from build123d import *

# Parameters (mm, degrees)
REVOLVE1_ANGLE     = 180
SKETCH3_R          = 1
CUT_EXTRUDE1_DEPTH = 2.5


with BuildPart() as part:
    # Sketch1 → Revolve1 (revolve)
    with BuildSketch(Plane(origin=(0, 0, 0), x_dir=(1, 0, 0), z_dir=(0, 1, 0))):
        with BuildLine():
            Line((0, 18.516950365), (120, 9.258475183))
            ThreePointArc((120, 9.258475183), (126.546730585, 6.546730585), (129.258475183, 0))
            Line((129.258475183, 0), (126, 0))
            ThreePointArc((126, 0), (124.242640687, 4.242640687), (120, 6))
            Line((120, 6), (0, 14))
            ThreePointArc((0, 14), (-9.899494937, 9.899494937), (-14, 0))
            Line((-14, 0), (-18.516950365, 0))
            ThreePointArc((-18.516950365, 0), (-13.09346117, 13.09346117), (0, 18.516950365))
        make_face()
    revolve(axis=Axis((-18.516950365, 0, 0), (1, 0, 0)), revolution_arc=REVOLVE1_ANGLE)

    # Sketch3 → Cut-Extrude1 (cut)
    with BuildSketch(Plane.XZ):
        with Locations(Location((-16, 0, 0), (0, 0, 270))):
            Circle(SKETCH3_R)
        with Locations(Location((0, 16, 0), (0, 0, 270))):
            Circle(SKETCH3_R)
        with Locations(Location((0, -16, 0), (0, 0, 270))):
            Circle(SKETCH3_R)
        with Locations(Location((127.5, 0, 0), (0, 0, 270))):
            Circle(SKETCH3_R)
    extrude(amount=-CUT_EXTRUDE1_DEPTH, mode=Mode.SUBTRACT)


solid = part.part
Can you work these out from the model? Positions are in its coordinate system, mm. A direction names the side the tool comes from. Give positions to 0.01 mm unless a question says otherwise; leave off trailing zeros. Loops run counter-clockwise (first coordinate to the right, second up) from the corner with the lowest first, then second, coordinate; pieces in that order, holes last. Notation, with made-up numbers: (16, -38.75) -> (50, -38.75) arc R24 ccw to (50, -20.75) -> close; hole circle Ø10 at (58.5, -22). An arc over 180 degrees is marked (long way). Return JSON: item names as keys, results as strings.
Q1. I want a section at B-B, the plane x = 15. List the corners of the cut face in (y, z) for me.
Checks:
{"outline": "(0, -17.36) arc R17.36 ccw to (0, 17.36) -> (0, 13) arc R13 cw to (0, -13) -> close"}
Q2. I want a section at A-A, the plane x = 87. List the corners of the cut face in (y, z) for me, then the cut area to 3 significant figures.
Checks:
{"outline": "(0, -11.8) arc R11.8 ccw to (0, 11.8) -> (0, 8.2) arc R8.2 cw to (0, -8.2) -> close", "area": "113 mm2"}
Q3. For pin 1 Ø1 at (x, y) = (80.5, 5) entering from +Z; pin 2 Ø3 at (y, z) = (6, -0.5) entering from +X; pin 3 Ø5 at (x, z) = (57, -14.5) entering from +Y, each with a flat end and sliding along its axis, tell me the tip position at first contact or that it passes through.
Checks:
{"pin 1": "stops at z = 11.46", "pin 2": "stops at x = 128.08", "pin 3": "stops at y = 7.46"}
Q4. On a 3-axis mill with a long thin cutter (end or side, diameter ignored), from which of +Z, -Z, +X, -X, +Y, -Y can I reach the whole of each face in a straight line? I mean faces 1 (the face through (59.16, 10.054, -0.221)), 2 (the face through (60.84, 13.82, -0.3)). Say none if no direction works.
Checks:
{"face 1": "-Y", "face 2": "+X, +Y"}
Q5. I need wall thicknesses on probe 1 along X at (y, z) = (0.75, 0); probe 2 along X at (y, z) = (1.35, 0); probe 3 along Z at (x, y) = (4.5, 1.75). Which ranges of each line are inside material? Lowest first, please.
Checks:
{"probe 1": "x = -18.5 to -17, -15 to -13.98, 125.95 to 126.5, 128.5 to 129.23", "probe 2": "x = -18.47 to -17, -15 to -13.93, 125.85 to 126.5, 128.5 to 129.16", "probe 3": "z = -18.09 to -13.59, 13.59 to 18.09"}
